Could you check a few things on this model? Use its own coordinates, in mm. Face numbers are marked on the shaded views. A direction names the side the tool comes from. Round coordinates to 2 decimals unless told otherwise and drop trailing zeros. Loops run counter-clockwise (first coordinate to the right, second up) from the corner with the lowest first, then second, coordinate; pieces in that order, holes last. Notation, with made-up numbers: (-29.5, 58) -> (-14.5, 58) arc R13 ccw to (-14.5, 67) -> close; hole circle Ø6 at (-35.5, 14.5). An arc over 180 degrees is marked (long way). Write each question's results on one line, items separated by ' | '.
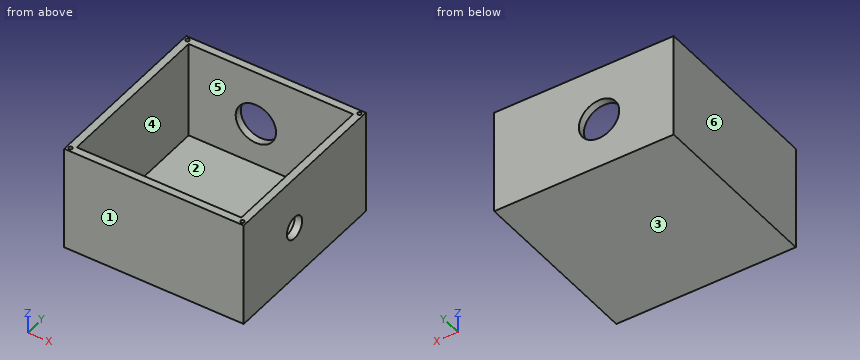
Autodesk Inventor part; units mm, degrees
ref_plane "YZ Plane" through (0, 0, 0) normal (1, 0, 0) x (0, 1, 0)
ref_plane "XZ Plane" through (0, 0, 0) normal (0, 1, 0) x (-1, 0, 0)
ref_plane "XY Plane" through (0, 0, 0) normal (0, 0, 1) x (1, 0, 0)
sketch "Sketch18" plane through (0, 0, 0) normal (0, 0, 1) x (1, 0, 0)
  line L0 (0, 0) -> (120, 0)
  line L1 (120, 0) -> (120, 120)
  line L2 (120, 120) -> (0, 120)
  line L3 (0, 120) -> (0, 0)
  dimension "d90" = 120
  dimension "d91" = 120
  dimension "d92" = 120
  dimension "d93" = 120
extrude "Extrusion4" add sketch "Sketch18" along normal blind 70
sketch "Sketch20" plane through (0, 0, 70) normal (0, 0, 1) x (1, 0, 0)
  point P0 (0, 0)
sketch "Sketch21" plane through (0, 0, 70) normal (0, 0, 1) x (1, 0, 0)
  line L0 (120, 120) -> (0, 120)
  line L1 (0, 120) -> (0, 115)
  line L2 (0, 120) -> (0, 0)
  line L3 (0, 115) -> (115, 115)
  line L4 (115, 115) -> (115, 5)
  line L5 (115, 5) -> (5, 5)
  line L6 (5, 5) -> (5, 115)
  dimension "d102" = 5
  dimension "d103" = 115
  dimension "d104" = 110
  dimension "d105" = 110
  dimension "d106" = 110
sketch "Sketch23" plane through (0, 0, 70) normal (0, 0, 1) x (1, 0, 0)
  line L0 (5.0371, 115.0535) -> (115.0371, 115.0535)
  line L1 (115.0371, 115.0535) -> (115.0371, 5.0535)
  line L2 (115.0371, 5.0535) -> (5.0371, 5.0535)
  line L3 (5.0371, 5.0535) -> (5.0371, 115.0535)
  line L4 (0, 0) -> (2.5, 0)
  line L5 (0, 0) -> (120, 0)
  line L6 (2.5, 0) -> (2.5, 2.5)
  circle A0 centre (2.5, 2.5) radius 1.25
  dimension "d108" = 110
  dimension "d109" = 110
  dimension "d110" = 110
  dimension "d143" = 2.5
  dimension "d144" = 2.5
  dimension "d145" = 2.5
extrude "Extrusion5" cut sketch "Sketch21" against normal blind 65
sketch "Sketch24" plane through (5, 115, 70) normal (0, -1, 0) x (1, 0, 0)
  point P0 (-5, -70)
sketch "Sketch25" plane through (0, 120, 0) normal (0, 1, 0) x (1, 0, 0)
  line L0 (0, 0) -> (120, 0)
  line L1 (0, 0) -> (50, 0)
  line L2 (50, 0) -> (50, -33.5)
  dimension "d113" = 50
  dimension "d114" = 33.5
sketch "Sketch26" plane through (0, 120, 0) normal (0, 1, 0) x (1, 0, 0)
  circle A0 centre (49.9198, -33.5778) radius 13.5
  point P0 (0, 0)
  dimension "d116" = 27
hole "Hole7" at (49.9198, 120, 33.5778) direction (0, -1, 0) diameter 27 depth 30
sketch "Sketch27" plane through (120, 0, 0) normal (1, 0, 0) x (0, 0, -1)
  line L0 (0, 0) -> (0, 50)
  line L1 (0, 120) -> (0, 0)
  line L2 (0, 50) -> (-35, 50)
  circle A0 centre (-35, 50) radius 7.5
  dimension "d124" = 50
  dimension "d125" = 35
  dimension "d126" = 15
hole "Hole8" at (120, 50, 35) direction (-1, 0, 0) diameter 15 depth 30
sketch "Sketch28" plane through (0, 0, 70) normal (0, 0, 1) x (1, 0, 0)
  line L0 (0, 120) -> (0, 0)
  line L1 (0, 120) -> (2.5, 120)
  line L2 (120, 120) -> (0, 120)
  line L3 (2.5, 120) -> (2.5, 117.5)
  dimension "d134" = 2.5
  dimension "d135" = 2.5
hole "Hole9" at (2.5, 117.5, 70) direction (0, 0, -1) diameter 2.5 depth 38.1 tip angle 118
hole "Hole10" at (2.5, 2.5, 70) direction (0, 0, -1) diameter 2.5 depth 38.1 tip angle 118
sketch "Sketch29" plane through (115, 5, 70) normal (-1, 0, 0) x (0, 0, 1)
  point P0 (-70, -5)
sketch "Sketch30" plane through (0, 0, 70) normal (0, 0, 1) x (1, 0, 0)
  line L0 (120, 120) -> (0, 120)
  line L1 (120, 120) -> (117.5, 120)
  line L2 (117.5, 120) -> (120, 120)
  point P0 (0, 0)
  dimension "d153" = 2.5
  dimension "d154" = 2.5
sketch "Sketch31" plane through (0, 0, 70) normal (0, 0, 1) x (1, 0, 0)
  line L0 (120, 120) -> (0, 120)
  line L1 (117.5038, 120) -> (120.0038, 120)
  line L2 (120.0038, 120) -> (120.0038, 117.5)
  line L3 (120.0038, 117.5) -> (117.5038, 117.5)
  point P0 (0, 0)
  dimension "d155" = 2.5
  dimension "d156" = 2.5
  dimension "d157" = 2.5
hole "Hole11" at (117.5038, 117.5, 70) direction (0, 0, -1) diameter 2.5 depth 38.1 tip angle 118
sketch "Sketch32" plane through (0, 0, 70) normal (0, 0, 1) x (1, 0, 0)
  line L0 (0, 0) -> (120, 0)
  line L1 (120, 0) -> (120, 2.5)
  line L2 (120, 0) -> (120, 120)
  line L3 (120, 2.5) -> (117.5, 2.5)
  dimension "d165" = 2.5
  dimension "d166" = 2.5
hole "Hole12" at (117.5, 2.5, 70) direction (0, 0, -1) diameter 2.5 depth 38.1 tip angle 118
properties part number "3d_enclosure_2_19_1"
1) I'm going to push a flat-ended pin straight in: pin 1 (6 mm diameter, centred on x = 103.5, y = 105.5, fed in from +Z). Where does the tip first touch, or does it pass through?
Model answer:
pin 1: stops at z = 5
2) I want a section at A-A, the plane z = 12. Write out the boundary of the cut face in (x, y).
Model answer:
outline: (0, 0) -> (120, 0) -> (120, 120) -> (0, 120) -> close; hole (5, 5) -> (115, 5) -> (115, 115) -> (5, 115) -> close
3) I need wall thicknesses on line 1 (X direction, y = 96, z = 16); line 2 (Z direction, x = 117, y = 50). Which ranges of each line are inside material? Lowest first, please.
Model answer:
line 1: x = 0 to 5, 115 to 120 | line 2: z = 0 to 27.5, 42.5 to 70
4) If we mould it in two halves opening along X, with no side actions, what happens to the marked faces 3, 4, 5 and 6? For each: released by +X, released by -X, zero draft, split by the parting line, or undercut.
Model answer:
face 3: zero draft | face 4: undercut | face 5: undercut | face 6: released by -X
5) I want a section at B-B, the plane y = 112. Write out the boundary of the cut face in (x, z).
Model answer:
outline: (0, 0) -> (120, 0) -> (120, 70) -> (115, 70) -> (115, 5) -> (5, 5) -> (5, 70) -> (0, 70) -> close
6) I want a section at D-D, the plane y = 50. Write out the boundary of the cut face in (x, z), plus the area to 4 significant figures.
Model answer:
outline: (0, 0) -> (120, 0) -> (120, 27.5) -> (115, 27.5) -> (115, 5) -> (5, 5) -> (5, 70) -> (0, 70) -> close; (115, 42.5) -> (120, 42.5) -> (120, 70) -> (115, 70) -> close | area: 1,175 mm2
7) For the marked faces 1 and 2, which set-ups out of +Z, -Z, +X, -X, +Y, -Y let a thin tool reach every point of the face, with its end or its side?
Model answer:
face 1: +Z, -Z, +X, -X, -Y | face 2: +Z
8) I want a section at C-C, the plane z = 35. Write out the boundary of the cut face in (x, y).
Model answer:
outline: (0, 0) -> (120, 0) -> (120, 42.5) -> (115, 42.5) -> (115, 5) -> (5, 5) -> (5, 115) -> (36.49, 115) -> (36.49, 120) -> (0, 120) -> close; (63.34, 115) -> (115, 115) -> (115, 57.5) -> (120, 57.5) -> (120, 120) -> (63.34, 120) -> close; hole circle Ø2.5 at (2.5, 2.5); hole circle Ø2.5 at (2.5, 117.5); hole circle Ø2.5 at (117.5, 2.5); hole circle Ø2.5 at (117.5, 117.5)
